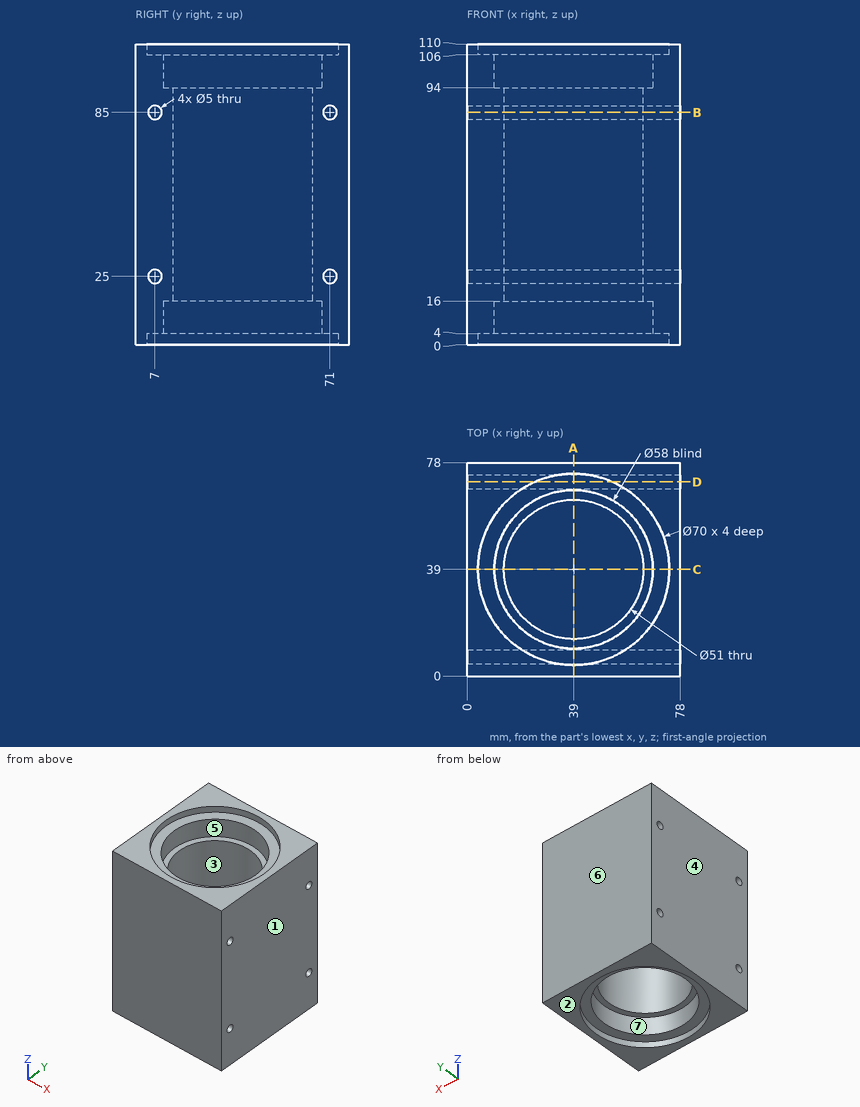
The figure shows three views and two pictorial views of one solid part (mm, origin at its lowest corner). Answer the questions. A direction names the side the tool comes from. Give positions to 0.01 mm unless a question says otherwise; leave off trailing zeros. Loops run counter-clockwise (first coordinate to the right, second up) from the corner with the lowest first, then second, coordinate; pieces in that order, holes last. Notation, with made-up numbers: (-1.5, 65.25) -> (6.5, 65.25) arc R6 cw to (6.5, 74.25) -> close; hole circle Ø4 at (10.5, 79). An arc over 180 degrees is marked (long way). Use a Markdown table: item, result. Add a question column.
1. Section A-A on x = 39 is taken. Determine the outline of the cut face in (y, z).
2. Section C-C on y = 39 is taken. Determine the outline of the cut face in (x, z).
3. Section D-D on y = 71 is taken. Determine the outline of the cut face in (x, z), and give its area (3 significant figures).
4. Section B-B on z = 85 is taken. Determine the outline of the cut face in (x, y), and give its area (3 significant figures).
5. Determine the mould class of the marked faces 1, 2, 3 and 4 for opening direction X: released by +X, released by -X, zero draft, split by the parting line, or undercut.
6. A flat-ended cylindrical pin translates along its axis: pin 1 Ø6 at (y, z) = (71, 85) entering from +X. Find the tip coordinate at first contact, or state that the pin passes through.
7. For the marked faces 5, 6 and 7, determine the directions among +Z, -Z, +X, -X, +Y, -Y from which every point of the face is accessible in a straight line to the end or side of a thin tool.
8. Find the intervals of material crossed by probe 1 along Z at (x, y) = (33, 71); probe 2 along Y at (x, z) = (39, 107.2); probe 3 along X at (y, z) = (62, 50.5), in increasing order.
Results below:
| question | item | result |
|---|---|---|
| 1 | outline | (0, 0) -> (4, 0) -> (4, 4) -> (10, 4) -> (10, 16) -> (13.5, 16) -> (13.5, 94) -> (10, 94) -> (10, 106) -> (4, 106) -> (4, 110) -> (0, 110) -> close; (64.5, 16) -> (68, 16) -> (68, 4) -> (74, 4) -> (74, 0) -> (78, 0) -> (78, 110) -> (74, 110) -> (74, 106) -> (68, 106) -> (68, 94) -> (64.5, 94) -> close; hole circle Ø5 at (7, 25); hole circle Ø5 at (7, 85); hole circle Ø5 at (71, 25); hole circle Ø5 at (71, 85) |
| 2 | outline | (0, 0) -> (4, 0) -> (4, 4) -> (10, 4) -> (10, 16) -> (13.5, 16) -> (13.5, 94) -> (10, 94) -> (10, 106) -> (4, 106) -> (4, 110) -> (0, 110) -> close; (64.5, 16) -> (68, 16) -> (68, 4) -> (74, 4) -> (74, 0) -> (78, 0) -> (78, 110) -> (74, 110) -> (74, 106) -> (68, 106) -> (68, 94) -> (64.5, 94) -> close |
| 3 | outline | (0, 0) -> (24.82, 0) -> (24.82, 4) -> (53.18, 4) -> (53.18, 0) -> (78, 0) -> (78, 22.5) -> (0, 22.5) -> close; (0, 27.5) -> (78, 27.5) -> (78, 82.5) -> (0, 82.5) -> close; (0, 87.5) -> (78, 87.5) -> (78, 110) -> (53.18, 110) -> (53.18, 106) -> (24.82, 106) -> (24.82, 110) -> (0, 110) -> close |
| 3 | area | 7,570 mm^2 |
| 4 | outline | (0, 0) -> (78, 0) -> (78, 4.5) -> (0, 4.5) -> close; (0, 9.5) -> (78, 9.5) -> (78, 68.5) -> (0, 68.5) -> close; (0, 73.5) -> (78, 73.5) -> (78, 78) -> (0, 78) -> close; hole circle Ø51 at (39, 39) |
| 4 | area | 3,260 mm^2 |
| 5 | face 1 | released by +X |
| 5 | face 2 | zero draft |
| 5 | face 3 | undercut |
| 5 | face 4 | released by -X |
| 6 | pin 1 | stops at x = 78 |
| 7 | face 5 | +Z |
| 7 | face 6 | +Z, -Z, +X, -X, +Y |
| 7 | face 7 | -Z |
| 8 | probe 1 | z = 4 to 22.5, 27.5 to 82.5, 87.5 to 106 |
| 8 | probe 2 | y = 0 to 4, 74 to 78 |
| 8 | probe 3 | x = 0 to 27.99, 50.01 to 78 |
